Design review of the part built by this model. Coordinates are the model's own, in mm. A direction names the side the tool comes from. Coordinates: 2 decimals unless noted, no trailing zeros. Write each loop counter-clockwise with the first axis right and the second up, starting at its lowest first coordinate (ties: lowest second). Pieces come first, ordered by that corner, then holes.
Q1. Machinability: for faces 1 (the flat face through (42, 33, -78.45)), 2 (the flat face through (127.1, 18, -40)), 3 (the flat face through (37, 32, -11.55)), which of the approach directions +Z, -Z, +X, -X, +Y, -Y give a long, thin tool a straight path to every point of the face, cutting with its end or side? Answer none if there is none.
Q2. Mouldability with a two-part tool opening along X and no side actions: class faces 4 (the flat face through (139, 16.45, -40)), 5 (the flat face through (123, 42, -56)), 6 (the flat face through (181.23, 32.54, -65.07)) as pulls with the +X half, pulls with the -X half, needs draft (parallel to the pull), parting line crosses it, or undercut.
Q3. For probe 1 along Y at (x, z) = (116, -80); probe 2 along Z at (x, y) = (146, 5); probe 3 along Z at (x, y) = (71, 36.5), list the stretches that pass through material, from the lowest coordinate up.
Q4. Take a section at A-A (x = 146.1). Give the boundary of the cut face in (y, z), and give its area (3 significant figures).
Q5. Insertion check: pin 1 (5 mm diameter, centred on x = 29.5, z = -57.5, fed in from -Y); pin 2 (5 mm diameter, centred on x = 117.5, z = -5.5, fed in from +Y); pin 3 (5 mm diameter, centred on x = 131.51, y = -65, fed in from -Z); pin 4 (5 mm diameter, centred on x = 168.5, y = -4.5, fed in from +Z). Each pin has a flat end and moves straight along its axis. Give the tip position at first contact, or say it passes through.
Q6. Take a section at C-C (y = 38.45). State how many separate pieces and enclosed holes the cut face has, and give its area (3 significant figures).
Q7. Take a section at B-B (x = 32). Give the boundary of the cut face in (y, z).
```python
from build123d import *

# Parameters (mm, degrees)
BOSS_EXTRUDE1_DEPTH  = 10
SKETCH2_W            = 9.45
SKETCH2_H            = 60
BOSS_EXTRUDE2_DEPTH  = 39.45
SKETCH3_W            = 24.96
SKETCH3_H            = 60
BOSS_EXTRUDE3_DEPTH  = 6.45
SKETCH4_W            = 9
SKETCH4_H            = 60
BOSS_EXTRUDE4_DEPTH  = 39.45
CUT_EXTRUDE1_REACH   = 209.197
SKETCH5_W            = 34
SKETCH5_H            = 28
CUT_EXTRUDE2_REACH   = 183.658
SKETCH7_W            = 76
SKETCH7_H            = 11.55
BOSS_EXTRUDE5_DEPTH  = 44.46
SKETCH8_W            = 76
SKETCH8_H            = 10
BOSS_EXTRUDE6_DEPTH  = 44.46
SKETCH9_W            = 10
SKETCH9_H            = 78.45
BOSS_EXTRUDE7_DEPTH  = 60
SKETCH10_W           = 2.5
SKETCH10_H           = 60
BOSS_EXTRUDE8_DEPTH  = 32.1
BOSS_EXTRUDE12_DEPTH = 10
CUT_EXTRUDE5_DEPTH   = 228.829497871
SKETCH17_W           = 10
SKETCH17_H           = 50
BOSS_EXTRUDE13_DEPTH = 80
SKETCH18_W           = 10
SKETCH18_H           = 50
BOSS_EXTRUDE14_DEPTH = 25
SKETCH19_R           = 3.5
CUT_EXTRUDE6_DEPTH   = 20
SKETCH20_W           = 27
SKETCH20_H           = 6
CUT_EXTRUDE7_DEPTH   = 10
SKETCH21_R           = 2.51
SKETCH21_R_2         = 19
CUT_EXTRUDE8_DEPTH   = 10
SKETCH22_R           = 3.1
CUT_EXTRUDE9_DEPTH   = 10
SKETCH23_R           = 3.1
CUT_EXTRUDE10_DEPTH  = 10
SKETCH24_R           = 10
BOSS_EXTRUDE15_DEPTH = 15
CUT_EXTRUDE11_START  = -8
SKETCH25_R           = 10
SKETCH25_R_2         = 7.5
CUT_EXTRUDE11_DEPTH  = 3
SKETCH26_R           = 10
BOSS_EXTRUDE16_DEPTH = 15
CUT_EXTRUDE12_START  = -8
SKETCH27_R           = 10
SKETCH27_R_2         = 7.5
CUT_EXTRUDE12_DEPTH  = 3


with BuildPart() as part:
    # Sketch1 → Boss-Extrude1 (new body)
    with BuildSketch(Plane(origin=(0, 0, 0), x_dir=(1, 0, 0), z_dir=(0, 1, 0))):
        Polygon((0, 0), (161.51, 0), (161.51, 70), (121.51, 70), (121.51, 120), (0, 120), align=None)
    extrude(amount=BOSS_EXTRUDE1_DEPTH)

    # Sketch2 → Boss-Extrude2 (add)
    with BuildSketch(Plane(origin=(0, 10, 0), x_dir=(1, 0, 0), z_dir=(0, 1, 0))):
        with Locations((156.785, 40)):
            Rectangle(SKETCH2_W, SKETCH2_H)
    extrude(amount=BOSS_EXTRUDE2_DEPTH)

    # Sketch3 → Boss-Extrude3 (add)
    with BuildSketch(Plane(origin=(0, 10, 0), x_dir=(1, 0, 0), z_dir=(0, 1, 0))):
        with Locations((139.58, 40)):
            Rectangle(SKETCH3_W, SKETCH3_H)
    extrude(amount=BOSS_EXTRUDE3_DEPTH)

    # Sketch4 → Boss-Extrude4 (add)
    with BuildSketch(Plane(origin=(0, 10, 0), x_dir=(1, 0, 0), z_dir=(0, 1, 0))):
        with Locations((122.6, 40)):
            Rectangle(SKETCH4_W, SKETCH4_H)
    extrude(amount=BOSS_EXTRUDE4_DEPTH)

    # Sketch5 → Cut-Extrude1 (cut, up to next)
    with BuildSketch(Plane(origin=(161.51, 0, 0), x_dir=(0, 0, -1), z_dir=(1, 0, 0)), mode=Mode.PRIVATE) as cut_extrude1_sk1:
        with Locations((40, 35.45)):
            Rectangle(SKETCH5_W, SKETCH5_H)
    cut_extrude1_tool1 = extrude(cut_extrude1_sk1.sketch, amount=-CUT_EXTRUDE1_REACH, mode=Mode.PRIVATE) & part.part
    add(cut_extrude1_tool1.solids().sort_by_distance((161.51, 35.45, -40))[0], mode=Mode.SUBTRACT)

    # Sketch6 → Cut-Extrude2 (cut, up to next)
    with BuildSketch(Plane(origin=(127.1, 0, 0), x_dir=(0, 0, -1), z_dir=(1, 0, 0)), mode=Mode.PRIVATE) as cut_extrude2_sk1:
        with BuildLine():
            Line((24, 49.45), (24, 34.24))
            ThreePointArc((24, 34.24), (40, 18.24), (56, 34.24))
            Line((56, 34.24), (56, 49.45))
            Line((56, 49.45), (24, 49.45))
        make_face()
    cut_extrude2_tool1 = extrude(cut_extrude2_sk1.sketch, amount=-CUT_EXTRUDE2_REACH, mode=Mode.PRIVATE) & part.part
    add(cut_extrude2_tool1.solids().sort_by_distance((127.1, 35.332249, -40))[0], mode=Mode.SUBTRACT)

    # Sketch7 → Boss-Extrude5 (add)
    with BuildSketch(Plane(origin=(0, 10, 0), x_dir=(1, 0, 0), z_dir=(0, 1, 0))):
        with Locations((38, 5.775)):
            Rectangle(SKETCH7_W, SKETCH7_H)
    extrude(amount=BOSS_EXTRUDE5_DEPTH)

    # Sketch8 → Boss-Extrude6 (add)
    with BuildSketch(Plane(origin=(0, 10, 0), x_dir=(1, 0, 0), z_dir=(0, 1, 0))):
        with Locations((38, 73.45)):
            Rectangle(SKETCH8_W, SKETCH8_H)
    extrude(amount=BOSS_EXTRUDE6_DEPTH)

    # Sketch9 → Boss-Extrude7 (add)
    with BuildSketch(Plane(origin=(0, 10, 0), x_dir=(1, 0, 0), z_dir=(0, 1, 0))):
        with Locations((81, 39.225)):
            Rectangle(SKETCH9_W, SKETCH9_H)
    extrude(amount=BOSS_EXTRUDE7_DEPTH)

    # Sketch10 → Boss-Extrude8 (add)
    with BuildSketch(Plane(origin=(86, 0, 0), x_dir=(0, 0, -1), z_dir=(1, 0, 0))):
        with Locations((68.75, 40)):
            Rectangle(SKETCH10_W, SKETCH10_H)
        with Locations((58.25, 40)):
            Rectangle(SKETCH10_W, SKETCH10_H)
        with Locations((21.75, 40)):
            Rectangle(SKETCH10_W, SKETCH10_H)
        with Locations((11.25, 40)):
            Rectangle(SKETCH10_W, SKETCH10_H)
    extrude(amount=BOSS_EXTRUDE8_DEPTH)

    # Sketch13 → Boss-Extrude12 (add)
    with BuildSketch(Plane(origin=(0, 0, -70), x_dir=(-1, 0, 0), z_dir=(0, 0, -1))):
        Polygon((-111.51, 0), (-161.51, 0), (-161.51, 49.45), (-201.51, 15.153701366), (-201.51, -24.846298634), (-161.51, -64.85), (-161.51, -80), (-111.51, -80), align=None)
    extrude(amount=-BOSS_EXTRUDE12_DEPTH)

    # Sketch16 → Cut-Extrude5 (cut, through all)
    with BuildSketch(Plane(origin=(0, 0, -70), x_dir=(-1, 0, 0), z_dir=(0, 0, -1))):
        Polygon((-86, 70), (-118.1, 70), (-118.1, 10), align=None)
    extrude(amount=-CUT_EXTRUDE5_DEPTH, mode=Mode.SUBTRACT)

    # Sketch17 → Boss-Extrude13 (add)
    with BuildSketch(Plane.XZ):
        with Locations((116.51, -95)):
            Rectangle(SKETCH17_W, SKETCH17_H)
    extrude(amount=BOSS_EXTRUDE13_DEPTH)

    # Sketch18 → Boss-Extrude14 (add)
    with BuildSketch(Plane(origin=(0, 10, 0), x_dir=(1, 0, 0), z_dir=(0, 1, 0))):
        with Locations((116.51, 95)):
            Rectangle(SKETCH18_W, SKETCH18_H)
    extrude(amount=BOSS_EXTRUDE14_DEPTH)

    # Sketch19 → Cut-Extrude6 (cut)
    with BuildSketch(Plane(origin=(0, 16.45, 0), x_dir=(1, 0, 0), z_dir=(0, 1, 0))):
        with Locations(Location((146.1, 62.98, 0), (0, 0, 270))):
            Circle(SKETCH19_R)
        with Locations(Location((133, 62.98, 0), (0, 0, 270))):
            Circle(SKETCH19_R)
        with Locations(Location((133, 16.98, 0), (0, 0, 270))):
            Circle(SKETCH19_R)
        with Locations(Location((146.1, 16.98, 0), (0, 0, 270))):
            Circle(SKETCH19_R)
    extrude(amount=-CUT_EXTRUDE6_DEPTH, mode=Mode.SUBTRACT)

    # Sketch20 → Cut-Extrude7 (cut)
    with BuildSketch(Plane.XY.offset(-60)):
        with Locations((139.6, -3)):
            Rectangle(SKETCH20_W, SKETCH20_H)
    extrude(amount=-CUT_EXTRUDE7_DEPTH, mode=Mode.SUBTRACT)

    # Sketch21 → Cut-Extrude8 (cut)
    with BuildSketch(Plane.ZY.offset(-76)):
        with Locations((-16.5, 61.95)):
            Circle(SKETCH21_R)
        with Locations((-63.5, 61.95)):
            Circle(SKETCH21_R)
        with Locations((-63.5, 14.95)):
            Circle(SKETCH21_R)
        with Locations((-16.5, 14.95)):
            Circle(SKETCH21_R)
        with Locations((-40, 38.45)):
            Circle(SKETCH21_R_2)
    extrude(amount=-CUT_EXTRUDE8_DEPTH, mode=Mode.SUBTRACT)

    # Sketch22 → Cut-Extrude9 (cut)
    with BuildSketch(Plane(origin=(0, 0, -70), x_dir=(-1, 0, 0), z_dir=(0, 0, -1))):
        with Locations((-131.51, -15)):
            Circle(SKETCH22_R)
        with Locations((-151.51, -15)):
            Circle(SKETCH22_R)
        with Locations((-151.51, -65)):
            Circle(SKETCH22_R)
        with Locations((-131.51, -65)):
            Circle(SKETCH22_R)
        with Locations((-191.51, 5.153701366)):
            Circle(SKETCH22_R)
        with Locations((-176.51, 5.153701366)):
            Circle(SKETCH22_R)
        with Locations((-176.51, -14.846298634)):
            Circle(SKETCH22_R)
        with Locations((-191.51, -14.846298634)):
            Circle(SKETCH22_R)
    extrude(amount=-CUT_EXTRUDE9_DEPTH, mode=Mode.SUBTRACT)

    # Sketch23 → Cut-Extrude10 (cut)
    with BuildSketch(Plane.ZY.offset(-111.51)):
        with Locations((-100, 25.93)):
            Circle(SKETCH23_R)
        with Locations((-80, 25.93)):
            Circle(SKETCH23_R)
        with Locations((-80, -15.01)):
            Circle(SKETCH23_R)
        with Locations((-100, -15.01)):
            Circle(SKETCH23_R)
        with Locations((-100, -65.01)):
            Circle(SKETCH23_R)
        with Locations((-80, -65.01)):
            Circle(SKETCH23_R)
    extrude(amount=-CUT_EXTRUDE10_DEPTH, mode=Mode.SUBTRACT)

    # Sketch24 → Boss-Extrude15 (add)
    with BuildSketch(Plane.XY.offset(-60)):
        with Locations(Location((126.51, -40, 0), (0, 0, 180))):
            Circle(SKETCH24_R)
    extrude(amount=BOSS_EXTRUDE15_DEPTH)

    # Sketch25 → Cut-Extrude11 (cut)
    with BuildSketch(Plane.XY.offset(-45).offset(CUT_EXTRUDE11_START)):
        with Locations(Location((126.51, -40, 0), (0, 0, 180))):
            Circle(SKETCH25_R)
        with Locations((126.51, -40)):
            Circle(SKETCH25_R_2, mode=Mode.SUBTRACT)
    extrude(amount=CUT_EXTRUDE11_DEPTH, mode=Mode.SUBTRACT)

    # Sketch26 → Boss-Extrude16 (add)
    with BuildSketch(Plane.ZY.offset(-111.51)):
        with Locations((-75, -40)):
            Circle(SKETCH26_R)
    extrude(amount=BOSS_EXTRUDE16_DEPTH)

    # Sketch27 → Cut-Extrude12 (cut)
    with BuildSketch(Plane.ZY.offset(-96.51).offset(CUT_EXTRUDE12_START)):
        with Locations((-75, -40)):
            Circle(SKETCH27_R)
        with Locations((-75, -40)):
            Circle(SKETCH27_R_2, mode=Mode.SUBTRACT)
    extrude(amount=CUT_EXTRUDE12_DEPTH, mode=Mode.SUBTRACT)


solid = part.part
```
Response:
1. face 1: -Z, -X, +Y
1. face 2: +Z, -Z, +Y
1. face 3: -X, +Y
2. face 4: undercut
2. face 5: needs draft
2. face 6: pulls with the +X half
3. probe 1: y = -80 to -68.11, -61.91 to -18.11, -11.91 to 22.83, 29.03 to 35
3. probe 2: z = -70 to -66.48, -59.48 to -20.48, -13.48 to 0
3. probe 3: z = -78.45 to -68.45, -11.55 to 0
4. outline: (-80, -70) - (-6, -70) - (-6, -60) - (-80, -60) - close; (0, -70) - (16.45, -70) - (16.45, -66.48) - (0, -66.48) - close; (0, -59.48) - (16.45, -59.48) - (16.45, -20.48) - (0, -20.48) - close; (0, -13.48) - (16.45, -13.48) - (16.45, -10) - (10, -10) - (10, 0) - (0, 0) - close
4. area: 1,600 mm2
5. pin 1: stops at y = 0
5. pin 2: stops at y = 10
5. pin 3: passes through
5. pin 4: stops at z = -60
6. separate pieces: 6
6. enclosed holes: 0
6. area: 2,840 mm2
7. outline: (0, -120) - (10, -120) - (10, -78.45) - (54.46, -78.45) - (54.46, -68.45) - (10, -68.45) - (10, -11.55) - (54.46, -11.55) - (54.46, 0) - (0, 0) - close
